Check sheet for the modelled part. Datum: model origin and axes. Units: mm. Coordinates: 2 decimals unless noted, no trailing zeros. Loops run counter-clockwise (first coordinate to the right, second up) from the corner with the lowest first, then second, coordinate; pieces in that order, holes last.
Autodesk Inventor part; units mm, degrees
ref_plane "YZ Plane" through (0, 0, 0) normal (1, 0, 0) x (0, 1, 0)
ref_plane "XZ Plane" through (0, 0, 0) normal (0, 1, 0) x (-1, 0, 0)
ref_plane "XY Plane" through (0, 0, 0) normal (0, 0, 1) x (1, 0, 0)
sketch "Sketch1" plane through (0, 0, 0) normal (0, 0, 1) x (1, 0, 0)
  line L0 (-54, -40.5) -> (54, -40.5)
  line L1 (54, -40.5) -> (54, 40.5)
  line L2 (54, 40.5) -> (-54, 40.5)
  line L3 (-54, 40.5) -> (-54, -40.5)
  point P0 (0, 0)
  dimension "d0" = 108
  dimension "d1" = 81
  dimension "d2" = 40.5
  dimension "d3" = 54
extrude "Extrusion1" add sketch "Sketch1" along normal blind 1.5875
hole "Hole2" at (50, -38, 1.5875) direction (0, 0, -1) diameter 2.6924 end through all
mirror "Mirror1" about plane through (0, 0, 0) normal (0, 1, 0) of "Hole2"
hole "Hole_audio" at (1.4, 28.5, 1.5875) direction (0, 0, -1) diameter 9.525 end through all
hole "Hole_mini_usb" [suppressed]
mirror "Mirror2" about plane through (0, 0, 0) normal (1, 0, 0) of "Hole2", "Mirror1"
hole "Hole5" at (0, -38, 1.5875) direction (0, 0, -1) diameter 2.6924 end through all
mirror "Mirror3" about plane through (0, 0, 0) normal (0, 1, 0) of "Hole5"
hole "Hole6" [suppressed]
mirror "Mirror4" [suppressed]
sketch "Sketch2" plane through (0, 0, 0) normal (0, 0, -1) x (-1, 0, 0)
  line L0 (-0.4125, -24.055) -> (-3.5875, -24.055)
  line L1 (-5.175, -25.6425) -> (-5.175, -31.3575)
  line L2 (-3.5875, -32.945) -> (-0.4125, -32.945)
  line L3 (1.175, -31.3575) -> (1.175, -25.6425)
  line L4 (-2, -22.5163) -> (-2, -34.6324)
  line L5 (-9.4902, -28.5) -> (-22.3716, -28.5)
  arc A0 (-0.4125, -32.945) -> (1.175, -31.3575) centre (-0.4125, -31.3575) ccw
  arc A1 (-5.175, -31.3575) -> (-3.5875, -32.945) centre (-3.5875, -31.3575) ccw
  arc A2 (-3.5875, -24.055) -> (-5.175, -25.6425) centre (-3.5875, -25.6425) ccw
  arc A3 (1.175, -25.6425) -> (-0.4125, -24.055) centre (-0.4125, -25.6425) ccw
  line L6 (54, -40.5) -> (-54, -40.5)
  point P0 (0, 0)
  point P1 (1.175, -24.055)
  point P2 (-5.175, -32.945)
  point P3 (1.175, -32.945)
  point P4 (-2, -28.5)
  dimension "d80" = 6.35
  dimension "d81" = 8.89
  dimension "d82" = 1.5875
  dimension "d85" = 12
  dimension "d87" = 2
extrude "cutout_mini_usb" cut sketch "Sketch2" against normal through all
sketch "Sketch4" plane through (0, 0, 1.5875) normal (0, 0, 1) x (1, 0, 0)
  line L0 (-54, -40.5) -> (-54, 40.5)
  line L1 (54, -40.5) -> (-54, -40.5)
  line L2 (54, 40.5) -> (54, -40.5)
  line L3 (-54, 40.5) -> (54, 40.5)
  line L4 (-53.878, -40.6622) -> (-54, 40.5) construction
  line L5 (-54, 40.5) -> (53.878, 40.6622) construction
  line L6 (53.878, 40.6622) -> (54, -40.5) construction
  line L7 (54, -40.5) -> (-53.878, -40.6622) construction
  point P0 (0, 0)
decal "Decal1"
sketch "Sketch5" plane through (0, 0, 0) normal (0, 0, -1) x (-1, 0, 0)
  line L0 (54, -40.5) -> (-54, -40.5)
  line L1 (54, 40.5) -> (54, -40.5)
  line L2 (-54, 40.5) -> (54, 40.5)
  line L3 (-54, -40.5) -> (-54, 40.5)
  line L4 (53.9396, 40.5804) -> (54, -40.5) construction
  line L5 (54, -40.5) -> (-53.9396, -40.5804) construction
  line L6 (-53.9396, -40.5804) -> (-54, 40.5) construction
  line L7 (-54, 40.5) -> (53.9396, 40.5804) construction
  point P0 (0, 0)
decal "Decal2"
properties part number "FOX-ME-119-05" material "FR4"
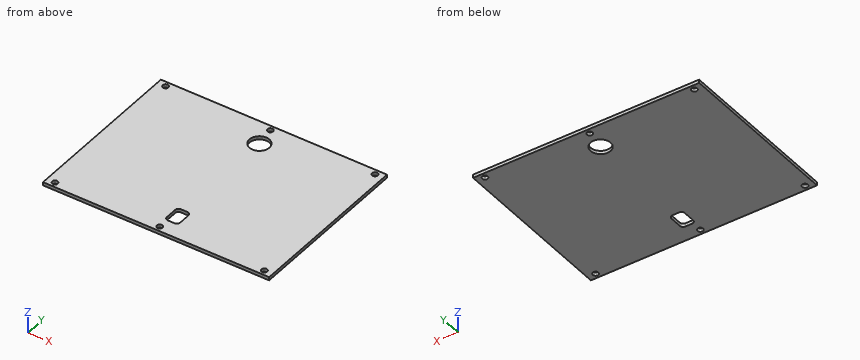
(1) Scan lines: line 1 along X through (y, z) = (38, 0.9); line 2 along Y through (x, z) = (1.4, 0.3) (1 decimal); line 3 along Y through (x, z) = (50, 0.65). Record each from-to range of solid material in increasing order.
(2) Section check C-C, the plane y = 28.5. Enter the section's corners in (x, z), plus the area to 3 significant figures.
(3) Section check A-A, the plane y = 38. Enter the section's corners in (x, z).
(4) Gauge pin test, flat end, axial feed: P1, Ø3.5, axis at x = 50, y = 38, coming from the +Z side. Record the tip position at first contact, or that the pin passes through.
(5) Section check B-B, the plane x = 50. Enter the section's corners in (y, z), plus the area to 3 significant figures.
(6) Section check D-D, the plane z = 1. Count the separate pieces of the cut face and the enclosed holes in it, plus the area to 3 significant figures.
Determined:
1. line 1: x = -54 to -51.35, -48.65 to -1.35, 1.35 to 48.65, 51.35 to 54
1. line 2: y = -40.5 to -32.9, -24.1 to 23.7, 33.3 to 40.5
1. line 3: y = -40.5 to -39.35, -36.65 to 36.65, 39.35 to 40.5
2. outline: (-54, 0) - (-3.36, 0) - (-3.36, 1.59) - (-54, 1.59) - close; (6.16, 0) - (54, 0) - (54, 1.59) - (6.16, 1.59) - close
2. area: 156 mm2
3. outline: (-54, 0) - (-51.35, 0) - (-51.35, 1.59) - (-54, 1.59) - close; (-48.65, 0) - (-1.35, 0) - (-1.35, 1.59) - (-48.65, 1.59) - close; (1.35, 0) - (48.65, 0) - (48.65, 1.59) - (1.35, 1.59) - close; (51.35, 0) - (54, 0) - (54, 1.59) - (51.35, 1.59) - close
4. P1: stops at z = 1.59
5. outline: (-40.5, 0) - (-39.35, 0) - (-39.35, 1.59) - (-40.5, 1.59) - close; (-36.65, 0) - (36.65, 0) - (36.65, 1.59) - (-36.65, 1.59) - close; (39.35, 0) - (40.5, 0) - (40.5, 1.59) - (39.35, 1.59) - close
5. area: 120 mm2
6. separate pieces: 1
6. enclosed holes: 8
6. area: 8,590 mm2
